The listing builds one solid part. Answer for the finished solid, in the listing's coordinates (mm). Face numbers are marked on the shaded views. A direction names the side the tool comes from. Give positions to 0.01 mm unless a question says otherwise; leave off trailing zeros. Order: outer loops, then holes, each group sorted by start corner. A loop starts at its lowest first (then second) coordinate and runs counter-clockwise, first axis right, second up. Notation, with made-up numbers: (49.25, 8) - (73.25, 8) arc R27 cw to (73.25, 43) - close; hole circle Ø5 at (84, 46). An arc over 180 degrees is marked (long way). Answer in a Markdown table with one row per item.
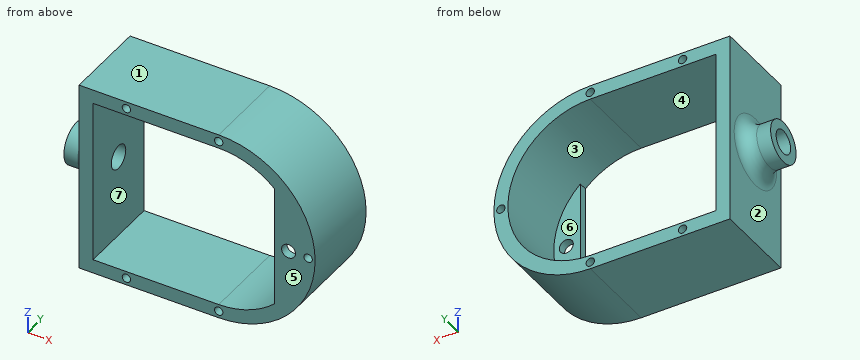
from build123d import *

# Parameters (mm, degrees)
SKETCH1_R           = 1.5
BOSS_EXTRUDE1_DEPTH = 30
SKETCH1_4_R         = 2.5
BOSS_EXTRUDE2_DEPTH = 3
SKETCH2_R           = 4.25
CUT_EXTRUDE1_DEPTH  = 3
BOSS_EXTRUDE3_START = 10
SKETCH3_R           = 7.5
SKETCH3_R_2         = 4.25
BOSS_EXTRUDE3_DEPTH = 10
FILLET1_R           = 5
SKETCH4_R           = 4.25
CUT_EXTRUDE2_DEPTH  = 10


with BuildPart() as part:
    # Sketch1 → Boss-Extrude1 (new body)
    with BuildSketch(Plane(origin=(0, 0, 0), x_dir=(1, 0, 0), z_dir=(0, 1, 0))):
        with BuildLine():
            Line((10, -34.5), (-40, -34.5))
            Line((-40, -34.5), (-40, 34.5))
            Line((-40, 34.5), (10, 34.5))
            ThreePointArc((10, 34.5), (44.5, 0), (10, -34.5))
        make_face()
        with Locations(Location((-23.050007367, 32, 0), (0, 0, 270))):
            Circle(SKETCH1_R, mode=Mode.SUBTRACT)
        with Locations(Location((-23.050007367, -32, 0), (0, 0, 270))):
            Circle(SKETCH1_R, mode=Mode.SUBTRACT)
        with Locations(Location((10, 32, 0), (0, 0, 270))):
            Circle(SKETCH1_R, mode=Mode.SUBTRACT)
        with Locations(Location((10, -32, 0), (0, 0, 270))):
            Circle(SKETCH1_R, mode=Mode.SUBTRACT)
        with Locations(Location((42, 0, 0), (0, 0, 270))):
            Circle(SKETCH1_R, mode=Mode.SUBTRACT)
        with BuildLine():
            Line((-35, 29.5), (10, 29.5))
            ThreePointArc((10, 29.5), (39.5, 0), (10, -29.5))
            Line((10, -29.5), (-35, -29.5))
            Line((-35, -29.5), (-35, 29.5))
        make_face(mode=Mode.SUBTRACT)
    extrude(amount=BOSS_EXTRUDE1_DEPTH)

    # Sketch1_4 → Boss-Extrude2 (add)
    with BuildSketch(Plane(origin=(0, 0, 0), x_dir=(1, 0, 0), z_dir=(0, 1, 0))):
        with BuildLine():
            ThreePointArc((30, -21.685248442), (39.5, 0), (30, 21.685248442))
            Line((30, 21.685248442), (30, 18.020023033))
            Line((30, 18.020023033), (30, -9.598736105))
            Line((30, -9.598736105), (30, -21.685248442))
        make_face()
        with Locations(Location((35, 0, 0), (0, 0, 270))):
            Circle(SKETCH1_4_R, mode=Mode.SUBTRACT)
    extrude(amount=BOSS_EXTRUDE2_DEPTH)

    # Sketch2 → Cut-Extrude1 (cut)
    with BuildSketch(Plane.ZY.offset(40)):
        with Locations((0, 15)):
            Circle(SKETCH2_R)
    extrude(amount=-CUT_EXTRUDE1_DEPTH, mode=Mode.SUBTRACT)

    # Sketch3 → Boss-Extrude3 (add)
    with BuildSketch(Plane.ZY.offset(40).offset(BOSS_EXTRUDE3_START)):
        with Locations((0, 15)):
            Circle(SKETCH3_R)
        with Locations((0, 15)):
            Circle(SKETCH3_R_2, mode=Mode.SUBTRACT)
    extrude(amount=-BOSS_EXTRUDE3_DEPTH)

    # Fillet1
    fillet1_edges = [part.edges().sort_by_distance(p)[0] for p in [
        (-40, 15, -7.5),
    ]]
    fillet(fillet1_edges, radius=FILLET1_R)

    # Sketch4 → Cut-Extrude2 (cut)
    with BuildSketch(Plane.ZY.offset(37)):
        with Locations((0, 15)):
            Circle(SKETCH4_R)
    extrude(amount=-CUT_EXTRUDE2_DEPTH, mode=Mode.SUBTRACT)


solid = part.part
Item 1: Find section D-D on z = -32. Write down the section's boundary in (x, y), then the cut area to 3 significant figures.
Answer block:
| item | result |
|---|---|
| outline | (-40, 0) - (-24.55, 0) - (-24.55, 30) - (-40, 30) - close; (-21.55, 0) - (8.5, 0) - (8.5, 30) - (-21.55, 30) - close; (11.5, 0) - (22.89, 0) - (22.89, 30) - (11.5, 30) - close |
| area | 1,710 mm² |
Item 2: Each of these flat-tipped pins is pushed along its axis until it touches: P1, Ø5, axis at y = 15, z = 0, coming from the -X side; P2, Ø2.5, axis at x = 42, z = 0, coming from the +Y side; P3, Ø6.5, axis at x = 35, z = 0, coming from the +Y side; P4, Ø0.9, axis at y = 1, z = -2, coming from the -X side. Where does it stop, or does it pass through?
Answer block:
| item | result |
|---|---|
| P1 | x = 39.39 |
| P2 | through |
| P3 | y = 3 |
| P4 | x = -40 |
Item 3: Which of the six approach directions +Z, -Z, +X, -X, +Y, -Y give full straight-line access (tool end or side, diameter ignored) to the marked faces 5, 6 and 7?
Answer block:
| item | result |
|---|---|
| face 5 | +Z, -Z, +X, -X, -Y |
| face 6 | +Y |
| face 7 | +Y, -Y |
Item 4: Determine the mould class of the marked faces 1, 2, 3 and 4 for opening direction X: pulls with the +X half, pulls with the -X half, needs draft (parallel to the pull), parting line crosses it, or undercut.
Answer block:
| item | result |
|---|---|
| face 1 | needs draft |
| face 2 | pulls with the -X half |
| face 3 | undercut |
| face 4 | undercut |
Item 5: Find section A-A on z = 0. Write down the section's boundary in (x, y).
Answer block:
| item | result |
|---|---|
| outline | (-50, 7.5) - (-45, 7.5) arc R5 cw to (-40, 2.5) - (-40, 0) - (-35, 0) - (-35, 10.75) - (-50, 10.75) - close; (-50, 19.25) - (-35, 19.25) - (-35, 30) - (-40, 30) - (-40, 27.5) arc R5 cw to (-45, 22.5) - (-50, 22.5) - close; (30, 0) - (32.5, 0) - (32.5, 3) - (30, 3) - close; (37.5, 0) - (40.5, 0) - (40.5, 30) - (39.5, 30) - (39.5, 3) - (37.5, 3) - close; (43.5, 0) - (44.5, 0) - (44.5, 30) - (43.5, 30) - close |
Item 6: Find section C-C on x = 35. Write down the section's boundary in (y, z).
Answer block:
| item | result |
|---|---|
| outline | (0, -23.77) - (30, -23.77) - (30, -15.66) - (3, -15.66) - (3, -2.5) - (0, -2.5) - close; (0, 2.5) - (3, 2.5) - (3, 15.66) - (30, 15.66) - (30, 23.77) - (0, 23.77) - close |
Item 7: Consider line 1 (X direction, y = 1.3, z = 0); line 2 (Z direction, x = -32, y = 27.5); line 3 (X direction, y = 24.25, z = 10). Determine where each line is inside the solid, lowest interval first.
Answer block:
| item | result |
|---|---|
| line 1 | -40 to -35, 30 to 32.5, 37.5 to 40.5, 43.5 to 44.5 |
| line 2 | -34.5 to -29.5, 29.5 to 34.5 |
| line 3 | -40 to -35, 37.75 to 43.02 |
Item 8: Find section B-B on y = 15. Write down the section's boundary in (x, z).
Answer block:
| item | result |
|---|---|
| outline | (-50, -7.5) - (-45, -7.5) arc R5 cw to (-40, -12.5) - (-40, -34.5) - (10, -34.5) arc R34.5 ccw to (10, 34.5) - (-40, 34.5) - (-40, 12.5) arc R5 cw to (-45, 7.5) - (-50, 7.5) - (-50, 4.25) - (-35, 4.25) - (-35, 29.5) - (10, 29.5) arc R29.5 cw to (10, -29.5) - (-35, -29.5) - (-35, -4.25) - (-50, -4.25) - close; hole circle Ø3 at (-23.05, -32); hole circle Ø3 at (-23.05, 32); hole circle Ø3 at (10, -32); hole circle Ø3 at (10, 32); hole circle Ø3 at (42, 0) |
